The figure shows three views and two pictorial views of one solid part (mm, origin at its lowest corner). Answer the questions. A direction names the side the tool comes from. Coordinates: 2 decimals unless noted, no trailing zeros. Write each loop counter-clockwise with the first axis right and the second up, starting at its lowest first coordinate (ties: lowest second). Pieces come first, ordered by that corner, then holes.
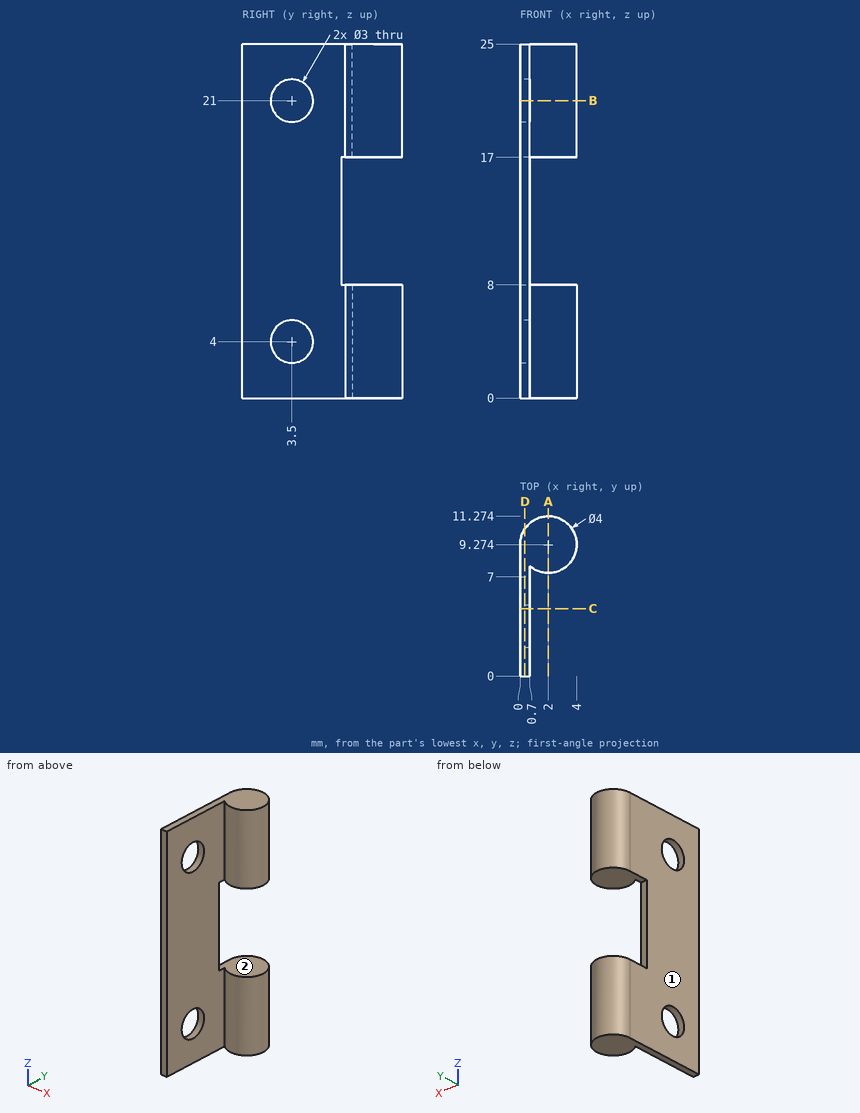
Item 1: The part is cut by section A-A (x = 2). Give the vertices of the cut face in (y, z).
Item 2: Find the intervals of material crossed by probe 1 along Z at (x, y) = (3.2, 8); probe 2 along X at (y, z) = (6, 6.75); probe 3 along Y at (x, z) = (0.45, 21) (1 decimal), in increasing order.
Item 3: Given pin 1 (2.5 mm diameter, centred on y = 3.5, z = 21, fed in from +X); pin 2 (5 mm diameter, centred on y = 3.5, z = 4, fed in from +X); pin 3 (0.6 mm diameter, centred on x = 0, z = 12.5, fed in from +Y), each flat-ended and moving along its own axis, determine where each tip first touches the part or whether it passes through.
Item 4: The part is cut by section D-D (x = 0.35). Give the vertices of the cut face in (y, z).
Item 5: For the marked faces 1 and 2, determine the directions among +Z, -Z, +X, -X, +Y, -Y from which every point of the face is accessible in a straight line to the end or side of a thin tool.
Item 6: The part is cut by section B-B (z = 21). Give the vertices of the cut face in (x, y).
Item 7: The part is cut by section C-C (y = 4.75). Give the vertices of the cut face in (x, z).
Answer:
1. outline: (7.27, 0) - (11.27, 0) - (11.27, 8) - (7.27, 8) - close; (7.27, 17) - (11.27, 17) - (11.27, 25) - (7.27, 25) - close
2. probe 1: z = 0 to 8, 17 to 25
2. probe 2: x = 0 to 0.7
2. probe 3: y = 0 to 2, 5 to 10.5
3. pin 1: passes through
3. pin 2: stops at x = 0.7
3. pin 3: stops at y = 7
4. outline: (0, 0) - (10.4, 0) - (10.4, 8) - (7, 8) - (7, 17) - (10.4, 17) - (10.4, 25) - (0, 25) - close; hole circle Ø3 at (3.5, 4); hole circle Ø3 at (3.5, 21)
5. face 1: +Z, -Z, -X, +Y, -Y
5. face 2: +X, -X, +Y
6. outline: (0, 0) - (0.7, 0) - (0.7, 2) - (0, 2) - close; (0, 5) - (0.7, 5) - (0.7, 7.75) arc R2 ccw (long way) to (0, 9.27) - close
7. outline: (0, 0) - (0.7, 0) - (0.7, 3.17) - (0, 3.17) - close; (0, 4.83) - (0.7, 4.83) - (0.7, 20.17) - (0, 20.17) - close; (0, 21.83) - (0.7, 21.83) - (0.7, 25) - (0, 25) - close
